from build123d import *

# Parameters (mm, degrees)
F0_R     = 222.25
F0_R_2   = 14.2875
F0_R_3   = 136.525
F1_DEPTH = 45.974
F2_W     = 45.974
F2_H     = 138.684
F2_H_2   = 21.59
F4_R     = 138.684
F5_DEPTH = 115.825
F6_R     = 161.925
F6_R_2   = 127.254
F7_DEPTH = 1.5875
F8_R     = 2.54
F9_DEPTH = 25.4


with BuildPart() as f1:
    # F0 (on Front) → F1 (new body)
    with BuildSketch(Plane.XZ):
        Circle(F0_R)
        with Locations((-37.7841181165, -189.9535891821)):
            Circle(F0_R_2, mode=Mode.SUBTRACT)
        with Locations((-107.6000648801, -161.0348771627)):
            Circle(F0_R_2, mode=Mode.SUBTRACT)
        with Locations((-161.0348771627, -107.6000648801)):
            Circle(F0_R_2, mode=Mode.SUBTRACT)
        with Locations((-189.9535891821, -37.7841181165)):
            Circle(F0_R_2, mode=Mode.SUBTRACT)
        with Locations((37.7841181165, -189.9535891821)):
            Circle(F0_R_2, mode=Mode.SUBTRACT)
        with Locations((107.6000648801, -161.0348771627)):
            Circle(F0_R_2, mode=Mode.SUBTRACT)
        with Locations((161.0348771627, -107.6000648801)):
            Circle(F0_R_2, mode=Mode.SUBTRACT)
        with Locations((189.9535891821, -37.7841181165)):
            Circle(F0_R_2, mode=Mode.SUBTRACT)
        with Locations((-189.9535891821, 37.7841181165)):
            Circle(F0_R_2, mode=Mode.SUBTRACT)
        with Locations((-161.0348771627, 107.6000648801)):
            Circle(F0_R_2, mode=Mode.SUBTRACT)
        with Locations((-107.6000648801, 161.0348771627)):
            Circle(F0_R_2, mode=Mode.SUBTRACT)
        with Locations((-37.7841181165, 189.9535891821)):
            Circle(F0_R_2, mode=Mode.SUBTRACT)
        Circle(F0_R_3, mode=Mode.SUBTRACT)
        with Locations((189.9535891821, 37.7841181165)):
            Circle(F0_R_2, mode=Mode.SUBTRACT)
        with Locations((161.0348771627, 107.6000648801)):
            Circle(F0_R_2, mode=Mode.SUBTRACT)
        with Locations((107.6000648801, 161.0348771627)):
            Circle(F0_R_2, mode=Mode.SUBTRACT)
        with Locations((37.7841181165, 189.9535891821)):
            Circle(F0_R_2, mode=Mode.SUBTRACT)
    extrude(amount=F1_DEPTH)

    # F2 (on Right) → F3 (revolve)
    with BuildSketch(Plane.YZ):
        with Locations((-22.987, 69.342)):
            Rectangle(F2_W, F2_H)
        with Locations((-22.987, 149.479)):
            Rectangle(F2_W, F2_H_2)
        Polygon((-115.824, 138.684), (-45.974, 138.684), (-45.974, 160.274), (-115.824, 151.3151675463), align=None)
    revolve(axis=Axis((0, -61.0863305628, 0), (0, -1, 0)))

    # F4 (on face) → F5 (cut, through all)
    with BuildSketch(Plane(origin=(0, 0, 0), x_dir=(-1, 0, 0), z_dir=(0, 1, 0))):
        Circle(F4_R)
    extrude(amount=-F5_DEPTH, mode=Mode.SUBTRACT)

    # F6 (on face) → F7 (join)
    with BuildSketch(Plane(origin=(0, 0, 0), x_dir=(-1, 0, 0), z_dir=(0, 1, 0))):
        Circle(F6_R)
        Circle(F6_R_2, mode=Mode.SUBTRACT)
    extrude(amount=F7_DEPTH)

    # F8
    f8_edges = [f1.edges().sort_by_distance(p)[0] for p in [
        (-222.25, 0, 0),
        (-222.25, -45.974, 0),
        (0, -45.974, -160.274),
    ]]
    fillet(f8_edges, radius=F8_R)

    # F9 (cut): a face of the model
    f9_faces = [f1.faces().sort_by_distance(p)[0] for p in [
        (134.7614241263, 0, 0),
    ]]
    extrude(f9_faces, amount=-F9_DEPTH, mode=Mode.SUBTRACT)


solid = f1.part
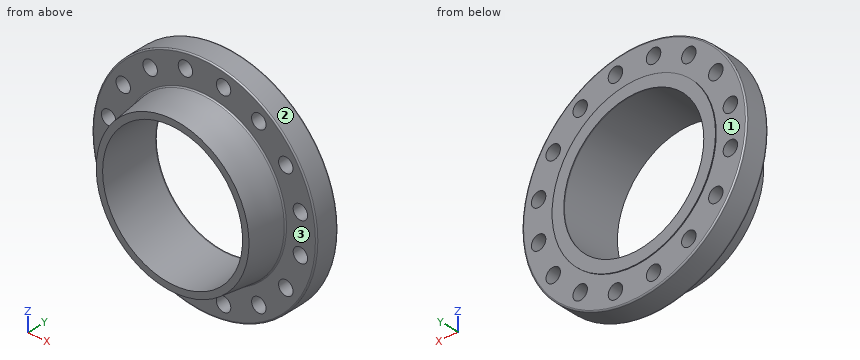
Can you work these out from the model? Positions are in its coordinate system, mm. Face numbers are marked on the shaded views. A direction names the side the tool comes from. Give positions to 0.01 mm unless a question says otherwise; leave off trailing zeros. Loops run counter-clockwise (first coordinate to the right, second up) from the corner with the lowest first, then second, coordinate; pieces in that order, holes last. Notation, with made-up numbers: M 74,34.5 L 106,34.5 A13 cw 106,54.5 Z; hole C -35,43.25 d6. An arc over 180 degrees is marked long. One line per item, written item: value. Start each with the question number.
1) If we section it at C-C, the plane y = -20.5: Give the number of separate pieces and of enclosed holes in the cut face, and give its area (3 significant figures).
2) If we section it at D-D, the plane y = -62.5: Write out the boundary of the cut face in (x, z), and give its area (3 significant figures).
3) If I drill on line 1 (X direction, y = -13, z = -157.5); line 2 (X direction, y = -44.5, z = 112.5); line 3 (X direction, y = -40, z = 180), over which ranges is the centre line in solid material (lowest first)? Write a range as [from, to].
4) I'm going to push flat-ended pins straight in: pin 1 (4 mm diameter, centred on x = 177.5, z = 26, fed in from -Y); pin 2 (5 mm diameter, centred on x = -75.5, y = -29.5, fed in from +Z); pin 3 (5 mm diameter, centred on x = 81.5, z = -162, fed in from +Y). Where does each tip first touch, or does it pass through?
5) On a 3-axis mill with a long thin cutter (end or side, diameter ignored), from which of +Z, -Z, +X, -X, +Y, -Y can I reach the whole of each face in a straight line? I mean the marked faces 1, 2 and 3. Say none if no direction works.
Completed:
1. separate pieces: 1
1. enclosed holes: 17
1. area: 84,500 mm^2
2. outline: C 0,0 d316.31; hole C 0,0 d277.37
2. area: 18,200 mm^2
3. line 1: x = [-156.81, -121.44], [-93.76, 93.76], [121.44, 156.81]
3. line 2: x = [-191.4, -174.46], [-147.61, -81.1], [81.1, 147.61], [174.46, 191.4]
3. line 3: x = [-130.37, -48.03], [-27.53, 27.53], [48.03, 130.37]
4. pin 1: stops at y = -45.97
4. pin 2: stops at z = 209.92
4. pin 3: stops at y = 0
5. face 1: +Y
5. face 2: +Y, -Y
5. face 3: -Y
